```python
from build123d import *

# Parameters (mm, degrees)
SKIZZE1_W                       = 24
SKIZZE1_H                       = 55
SKIZZE1_W_2                     = 12
SKIZZE1_H_2                     = 3.5
AUFSATZ_LINEAR_AUSTRAGEN1_DEPTH = 4
SKIZZE3_W                       = 20
SKIZZE3_H                       = 45
AUFSATZ_LINEAR_AUSTRAGEN3_DEPTH = 4
SCHNITT_LINEAR_AUSTRAGEN1_REACH = 6
SKIZZE4_R                       = 0.5


with BuildPart() as part:
    # Skizze1 → Aufsatz-Linear austragen1 (new body)
    with BuildSketch(Plane.XY):
        with Locations((12, 27.5)):
            Rectangle(SKIZZE1_W, SKIZZE1_H)
        with Locations((12, 47.25)):
            Rectangle(SKIZZE1_W_2, SKIZZE1_H_2, mode=Mode.SUBTRACT)
    extrude(amount=AUFSATZ_LINEAR_AUSTRAGEN1_DEPTH)

    # Skizze3 → Aufsatz-Linear austragen3 (add)
    with BuildSketch(Plane.XY.offset(4)):
        with Locations((34, 32.5)):
            Rectangle(SKIZZE3_W, SKIZZE3_H)
    extrude(amount=-AUFSATZ_LINEAR_AUSTRAGEN3_DEPTH)

    # Skizze4 → Schnitt-Linear austragen1 (cut, up to next)
    with BuildSketch(Plane.XY.offset(4), mode=Mode.PRIVATE) as schnitt_linear_austragen1_sk1:
        with Locations((30.6, 37.377592673)):
            Circle(SKIZZE4_R)
    schnitt_linear_austragen1_tool1 = extrude(schnitt_linear_austragen1_sk1.sketch, amount=-SCHNITT_LINEAR_AUSTRAGEN1_REACH, mode=Mode.PRIVATE) & part.part
    add(schnitt_linear_austragen1_tool1.solids().sort_by_distance((30.6, 37.377593, 4))[0], mode=Mode.SUBTRACT)


solid = part.part
```
CAD build for the part. Positions are in the model's coordinates, mm. A direction names the side the tool comes from. Round coordinates to 2 decimals unless told otherwise and drop trailing zeros. Order: outer loops, then holes, each group sorted by start corner. A loop starts at its lowest first (then second) coordinate and runs counter-clockwise, first axis right, second up.
Q1. Wall check: L1, parallel to Y at x = 30.6, z = 0.95; L2, parallel to X at y = 48, z = 3.3; L3, parallel to Y at x = 33.5, z = 2.6. Give the ranges that are in metal, low to high.
Q2. Which spindle directions (+Z, -Z, +X, -X, +Y, -Y) get a long thin tool onto all of the face, cutting with end or side? Do faces 1 (the flat face through (22, 28, 4)), 2 (the flat face through (24, 5, 2)), 3 (the flat face through (12, 49, 2)). Say none if no direction does.
Q3. Slice it at B-B (z = 2.6). Write the cut outline in (x, y).
Q4. Two-plate mould, pull along X, no slides. Class faces 4 (the flat face through (22, 55, 2)), 5 (the flat face through (6, 47, 2)), 6 (the flat face through (44, 32, 2)), 7 (the flat face through (0, 27, 2)): pulls with the +X half, pulls with the -X half, needs draft (parallel to the pull), parting line crosses it, or undercut.
Q5. Slice it at C-C (x = 33). Write the cut outline in (y, z).
Q6. Drop flat-ended pins along their axis: pin 1 (1.8 mm diameter, centred on y = 46.5, z = 2.5, fed in from -X); pin 2 (1 mm diameter, centred on y = 9, z = 2, fed in from +X); pin 3 (1.2 mm diameter, centred on x = 38, z = 1.5, fed in from -Y). Give the stop position or say it passes through.
Q7. Slice it at A-A (x = 9). Write the cut outline in (y, z).
Results below:
1. L1: y = 10 to 36.88, 37.88 to 55
1. L2: x = 0 to 6, 18 to 44
1. L3: y = 10 to 55
2. face 1: +Z, +X, -X, +Y, -Y
2. face 2: +Z, -Z, +X, -Y
2. face 3: +Z, -Z
3. outline: (0, 0) - (24, 0) - (24, 10) - (44, 10) - (44, 55) - (0, 55) - close; hole (6, 45.5) - (18, 45.5) - (18, 49) - (6, 49) - close; hole circle Ø1 at (30.6, 37.38)
4. face 4: needs draft
4. face 5: undercut
4. face 6: pulls with the +X half
4. face 7: pulls with the -X half
5. outline: (10, 0) - (55, 0) - (55, 4) - (10, 4) - close
6. pin 1: stops at x = 0
6. pin 2: stops at x = 24
6. pin 3: stops at y = 10
7. outline: (0, 0) - (45.5, 0) - (45.5, 4) - (0, 4) - close; (49, 0) - (55, 0) - (55, 4) - (49, 4) - close
